Autodesk Inventor part; units mm, degrees
ref_plane "YZ Plane" through (0, 0, 0) normal (1, 0, 0) x (0, 1, 0)
ref_plane "XZ Plane" through (0, 0, 0) normal (0, 1, 0) x (-1, 0, 0)
ref_plane "XY Plane" through (0, 0, 0) normal (0, 0, 1) x (1, 0, 0)
sketch "Esquisse1" plane through (0, 0, 0) normal (0, 1, 0) x (-1, 0, 0)
  line L0 (0, 0) -> (30, 0)
  line L1 (30, 0) -> (30, -23)
  line L2 (28, -25) -> (2, -25)
  line L3 (0, -23) -> (0, 0)
  circle A0 centre (15, -12.5) radius 8.25
  line L4 (30, -23) -> (28, -25)
  line L5 (2, -25) -> (0, -23)
  point P0 (0, 0)
  point P1 (30, -25)
  point P2 (0, -25)
  point P3 (11.5, 0)
  point P4 (30, -4)
  point P5 (21, 0)
  point P6 (0, -2)
  point P7 (2, 0)
  dimension "d0" = 25
  dimension "d1" = 30
  dimension "d2" = 16.5
  dimension "d3" = 15
  dimension "d11" = 2
  dimension "d12" = 2
  dimension "d13" = 2
  dimension "d14" = 2
  dimension "d47" = 12.5
extrude "Extrusion1" add sketch "Esquisse1" along normal blind 3.5
sketch "Esquisse2" plane through (0, 3.5, 0) normal (0, 1, 0) x (1, 0, 0)
  circle A0 centre (-15, 12.5) radius 8.25 construction
  circle A1 centre (-15, 12.5) radius 10.8894 construction
  line L0 (-22.7, 4.8) -> (-22.7, 20.2) construction
  line L1 (-22.7, 20.2) -> (-7.3, 20.2) construction
  line L2 (-7.3, 20.2) -> (-7.3, 4.8) construction
  line L3 (-7.3, 4.8) -> (-22.7, 4.8) construction
  point P0 (0, 0)
  dimension "d19" = 15.4
  dimension "d20" = 15.4
hole "Perçage1" at (-22.7, 3.5, -4.8) at (-22.7, 3.5, -20.2) at (-7.3, 3.5, -20.2) at (-7.3, 3.5, -4.8) direction (0, -1, 0) diameter 2.4 end through all counterbore diameter 4.4 counterbore depth 2
sketch "Esquisse3" plane through (-30, 0, 0) normal (0, 0, 1) x (1, 0, 0)
  line L0 (0, 3.5) -> (30, 3.5)
  line L1 (0, 3.5) -> (30, 3.5)
  line L2 (30, 3.5) -> (30, -26.5)
  line L3 (30, -26.5) -> (0, -26.5)
  line L4 (0, -26.5) -> (0, 3.5)
  point P0 (30, 0)
  point P1 (30, 3.5)
  dimension "d29" = 30
  dimension "d48" = 30
  dimension "d49" = 30
extrude "Extrusion2" add sketch "Esquisse3" along normal blind 5
sketch "Esquisse5" plane through (-30, 0, 0) normal (0, 0, -1) x (-1, 0, 0)
  line L0 (-5, -5) -> (-25, -5) construction
  line L1 (-25, -5) -> (-25, -20) construction
  line L2 (-25, -20) -> (-5, -20) construction
  line L3 (-5, -20) -> (-5, -5) construction
  line L4 (-28, 0) -> (-2, 0) construction
  line L5 (0, 0) -> (0, -23) construction
  point P0 (-30, 0)
  point P1 (0, -21)
  dimension "d36" = 15
  dimension "d37" = 20
  dimension "d38" = 5
  dimension "d39" = 5
hole "Perçage2" at (-25, -5, 0) at (-25, -20, 0) at (-5, -20, 0) at (-5, -5, 0) direction (0, 0, 1) diameter 3.4 end through all counterbore diameter 6.5 counterbore depth 3
sketch "Esquisse6" plane through (0, 0, -23) normal (1, 0, 0) x (0, 0, -1)
  line L0 (0, 3.5) -> (-28, 3.5)
  line L1 (-28, 3.5) -> (-38, 3.5)
  line L2 (-38, 3.5) -> (-38, -26.5)
  line L3 (-38, -26.5) -> (-28, -26.5)
  line L4 (-28, 3.5) -> (0, 3.5)
  line L5 (0, 3.5) -> (0, 0)
  line L6 (-23, -26.5) -> (-23, 0)
  line L7 (0, 0) -> (-23, -26.5)
  line L8 (-23, -26.5) -> (-28.3834, -26.5)
  dimension "d53" = 30
  dimension "d54" = 10
  dimension "d55" = 10
extrude "Extrusion4" add sketch "Esquisse6" along normal blind 2
equation "\"d3\" = 0.5 * d1"
equation "\"d47\" = 0.5 * d0"
equation "\"d20\" = d19"
equation "\"d48\" = d49"
equation "\"d55\" = d54"
properties part number "support nema8_gauche"
Source: CAD feature listing. Evaluate the final solid. Frame: model axes, mm. A direction names the side the tool comes from. Give positions to 0.01 mm unless a question says otherwise; leave off trailing zeros. Write each loop counter-clockwise with the first axis right and the second up, starting at its lowest first coordinate (ties: lowest second). Pieces come first, ordered by that corner, then holes. Notation, with made-up numbers: (20.25, -12.5) - (69.25, -12.5) arc R24 ccw to (69.25, 19.5) - close; hole circle Ø10 at (8, -35.75). An arc over 180 degrees is marked (long way). Write item = value, one per line. Start each with the question number.
Q1. Cut plane B-B, the plane y = -20.25. Return loops of the section in (x, z), then the cut area to 3 significant figures.
Q2. Pin query (flat end, axial travel): pin 1 Ø8.5 at (x, y) = (-25, -5) entering from -Z; pin 2 Ø1.6 at (x, y) = (1.5, 2.5) entering from -Z; pin 3 Ø1.5 at (x, y) = (-3, -4.5) entering from -Z. Return the tip coordinate at first contact, or that it passes through.
Q3. Cut plane A-A, the plane x = -15. Return loops of the section in (y, z).
Q4. Reachability of faces 1 (the flat face through (-3.6, -3.6, 3)), 2 (the flat face through (-11, 3.5, -5)), 3 (the cylindrical face through (-21.361, 2.486, -21.946)), 4 (the flat face through (-15, -11, 5)), 5 (the flat face through (2, -8, 0)) from +Z, -Z, +X, -X, +Y, -Y: full face, straight path, thin tool, end or side. Return the list, or none.
Q5. Material intervals for probe 1 along X at (y, z) = (-20, 1.9); probe 2 along Y at (x, z) = (-5, 2); probe 3 along X at (y, z) = (-20, 3.7), sorted ascending.
Q6. Cut plane D-D, the plane z = -20.2. Return loops of the section in (x, y), then the cut area to 3 significant figures.
Q7. Cut plane C-C, the plane x = -7.3. Give the number of separate pieces and of enclosed holes in the cut face, then the cut area to 3 significant figures.
Q8. Draft query along Z for faces 6 (the flat face through (-12, -26.5, 3)), 7 (the flat face through (0.986, -13.064, -11.661)), 8 (the cylindrical face through (-18.807, 1.726, -5.181)). Return one class per face: +Z half, -Z half, draft (parallel to the pull), parting line (faces both ways), or undercut.
Computed values:
q1.outline = (-30, 0) - (-28.24, 0) - (-28.24, 3) - (-26.68, 3) - (-26.68, 5) - (-30, 5) - close; (-23.32, 3) - (-21.76, 3) - (-21.76, 0) - (-8.24, 0) - (-8.24, 3) - (-6.68, 3) - (-6.68, 5) - (-23.32, 5) - close; (-3.32, 3) - (-1.76, 3) - (-1.76, 0) - (0, 0) - (0, -5.42) - (2, -5.42) - (2, 15) - (0, 15) - (0, 5) - (-3.32, 5) - close
q1.area = 139 mm²
q2.pin_1 = 0
q2.pin_2 = -23
q2.pin_3 = 3
q3.outline = (-26.5, 0) - (0, 0) - (0, -4.25) - (3.5, -4.25) - (3.5, 5) - (-26.5, 5) - close; (0, -25) - (3.5, -25) - (3.5, -20.75) - (0, -20.75) - close
q4.face_1 = -Z
q4.face_2 = +Z, -Z, +X, -X, +Y
q4.face_3 = +Y
q4.face_4 = +Z, -X, +Y, -Y
q4.face_5 = +Z, -Z, +X, +Y, -Y
q5.probe_1 = -30 to -28.25, -21.75 to -8.25, -1.75 to 2
q5.probe_2 = -26.5 to -23.25, -16.75 to -8.25, -1.75 to 3.5
q5.probe_3 = -30 to -26.7, -23.3 to -6.7, -3.3 to 2
q6.outline = (-30, 0) - (-23.9, 0) - (-23.9, 1.5) - (-24.9, 1.5) - (-24.9, 3.5) - (-30, 3.5) - close; (-21.5, 0) - (-17.96, 0) - (-17.96, 3.5) - (-20.5, 3.5) - (-20.5, 1.5) - (-21.5, 1.5) - close; (-12.04, 0) - (-8.5, 0) - (-8.5, 1.5) - (-9.5, 1.5) - (-9.5, 3.5) - (-12.04, 3.5) - close; (-6.1, 0) - (0, 0) - (0, -3.23) - (2, -3.23) - (2, 3.5) - (-5.1, 3.5) - (-5.1, 1.5) - (-6.1, 1.5) - close
q6.area = 72.9 mm²
q7.separate_pieces = 4
q7.enclosed_holes = 0
q7.area = 164 mm²
q8.face_6 = draft
q8.face_7 = -Z half
q8.face_8 = undercut
